Can you work these out from the drawing? Everything is in mm from the part's minimum corner. A direction names the side the tool comes from. Round coordinates to 2 decimals unless told otherwise and drop trailing zeros. Order: outer loops, then holes, each group sorted by start corner. A loop starts at its lowest first (then second) coordinate and runs counter-clockwise, first axis right, second up. Notation, with made-up numbers: (19.5, -33.75) -> (38.5, -33.75) arc R22 cw to (38.5, 0.25) -> close; hole circle Ø4 at (2, 72.25). An arc over 180 degrees is marked (long way). One line per item, written item: value.
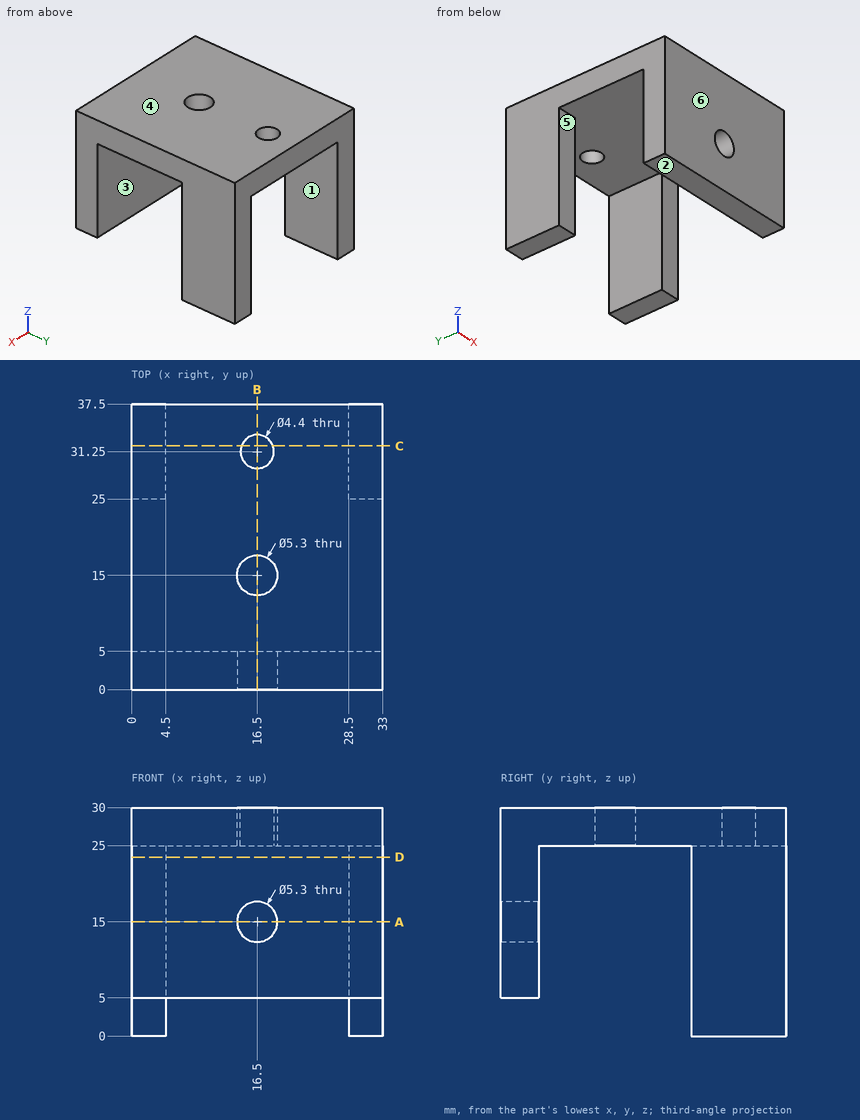
Q1. For P1, Ø4, axis at x = 17.5, y = 26.5, coming from the -Z side; P2, Ø1.5, axis at x = 22, y = 2, coming from the -Z side; P3, Ø2, axis at x = 9, z = 6, coming from the +Y side, each with a flat end and sliding along its axis, tell me the tip position at first contact or that it passes through.
Answers:
P1: z = 25
P2: z = 5
P3: y = 5
Q2. If we mould it in two halves opening along Y, with no side actions, what happens to the marked faces 4, 5 and 6? For each: pulls with the +Y half, pulls with the -Y half, needs draft (parallel to the pull), parting line crosses it, or undercut.
Answers:
face 4: needs draft
face 5: undercut
face 6: pulls with the -Y half
Q3. I want a section at D-D on z = 23.5. Write out the boundary of the cut face in (x, y).
Answers:
outline: (0, 0) -> (33, 0) -> (33, 5) -> (0, 5) -> close; (0, 25) -> (4.5, 25) -> (4.5, 37.5) -> (0, 37.5) -> close; (28.5, 25) -> (33, 25) -> (33, 37.5) -> (28.5, 37.5) -> close
Q4. I want a section at A-A on z = 15. Write out the boundary of the cut face in (x, y).
Answers:
outline: (0, 0) -> (13.85, 0) -> (13.85, 5) -> (0, 5) -> close; (0, 25) -> (4.5, 25) -> (4.5, 37.5) -> (0, 37.5) -> close; (19.15, 0) -> (33, 0) -> (33, 5) -> (19.15, 5) -> close; (28.5, 25) -> (33, 25) -> (33, 37.5) -> (28.5, 37.5) -> close
Q5. I need wall thicknesses on line 1 along Y through (x, z) = (16.5, 28.95); line 2 along X through (y, z) = (31, 12.5); line 3 along Y through (x, z) = (30, 20.5). Which ranges of each line are inside material? Lowest first, please.
Answers:
line 1: 0 to 12.35, 17.65 to 29.05, 33.45 to 37.5
line 2: 0 to 4.5, 28.5 to 33
line 3: 0 to 5, 25 to 37.5
Q6. I want a section at B-B on x = 16.5. Write out the boundary of the cut face in (y, z).
Answers:
outline: (0, 5) -> (5, 5) -> (5, 12.35) -> (0, 12.35) -> close; (0, 17.65) -> (5, 17.65) -> (5, 25) -> (12.35, 25) -> (12.35, 30) -> (0, 30) -> close; (17.65, 25) -> (29.05, 25) -> (29.05, 30) -> (17.65, 30) -> close; (33.45, 25) -> (37.5, 25) -> (37.5, 30) -> (33.45, 30) -> close
Q7. I want a section at C-C on y = 32. Write out the boundary of the cut face in (x, z).
Answers:
outline: (0, 0) -> (4.5, 0) -> (4.5, 25) -> (14.43, 25) -> (14.43, 30) -> (0, 30) -> close; (18.57, 25) -> (28.5, 25) -> (28.5, 0) -> (33, 0) -> (33, 30) -> (18.57, 30) -> close
Q8. Which directions (+Z, -Z, +X, -X, +Y, -Y) give clear straight access to the entire face, cutting with the end or side of a thin tool? Please do the marked faces 1, 2 and 3.
Answers:
face 1: -Z, +Y
face 2: -Z, +X, -X, -Y
face 3: -Z, +X, -X
